```python
from build123d import *

# Parameters (mm, degrees)
BOSS_EXTRUDE2_DEPTH = 3.175
FILLET1_R           = 12.7


with BuildPart() as part:
    # Sketch2 → Boss-Extrude2 (new body)
    with BuildSketch(Plane(origin=(125.924984682, -11.700540008, 0), x_dir=(0, 0, -1), z_dir=(0.9957109910599374, -0.0925182267579596, 0))):
        Polygon((-1098.963689663, 120.858697524), (-1344.041321718, 121.265601845), (-1344.041321718, 447.57468292), (-948.211534765, 482.774987334), align=None)
    extrude(amount=BOSS_EXTRUDE2_DEPTH)

    # Fillet1
    fillet1_edges = [part.edges().sort_by_distance(p)[0] for p in [
        (138.687308264, 108.492920797, 1098.963689663),
        (138.72495433, 108.898079901, 1344.041321718),
        (168.914491886, 433.807618411, 1344.041321718),
        (172.171161632, 468.856948404, 948.211534765),
    ]]
    fillet(fillet1_edges, radius=FILLET1_R)


solid = part.part
```
Input: part model. Units: mm. Frame: model coordinates. Give positions to 0.01 mm unless a question says otherwise; leave off trailing zeros. Order: outer loops, then holes, each group sorted by start corner. A loop starts at its lowest first (then second) coordinate and runs counter-clockwise, first axis right, second up. Notation, with made-up numbers: (4, 89) - (30, 89) arc R7 ccw to (30, 99) - close; hole circle Ø2 at (-7.5, -32.5). An arc over 180 degrees is marked (long way). Use a Markdown table: item, result.
(1) Section query A-A (x = 157). Output: boundary loops of the cut face in (y, z), then the cut area to 3 significant figures.
Computed values:
| item | result |
|---|---|
| outline | (288.42, 1023.63) - (322.74, 1009.4) - (322.74, 1344.04) - (288.42, 1344.04) - close |
| area | 11,200 mm2 |
(2) Line query: line 1 (X direction, y = 187, z = 1148.5); line 2 (X direction, y = 330, z = 1017); line 3 (Z direction, x = 161.5, y = 342). Output: solid intervals per line, ascending. Write a range as from..to.
Computed values:
| item | result |
|---|---|
| line 1 | x = 144.39..147.58 |
| line 2 | x = 157.67..160.86 |
| line 3 | z = 1001.24..1344.04 |
(3) Pin query (flat end, axial travel): pin 1 (3 mm diameter, centred on y = 309.5, z = 1043, fed in from +X); pin 2 (8 mm diameter, centred on x = 144.5, z = 1034.5, fed in from +Y); pin 3 (3 mm diameter, centred on y = 227.5, z = 1129, fed in from -X). Return the tip coordinate at first contact, or that it passes through.
Computed values:
| item | result |
|---|---|
| pin 1 | stops at x = 159.1 |
| pin 2 | passes through |
| pin 3 | stops at x = 148.01 |
(4) Section query B-B (z = 1310.5). Output: boundary loops of the cut face in (x, y).
Computed values:
| item | result |
|---|---|
| outline | (137.14, 108.99) - (140.3, 108.7) - (170.77, 436.63) - (167.61, 436.92) - close |
